from build123d import *

# Parameters (mm, degrees)
EXTRUDE_1_DEPTH     = 200
SKETCH_2_W          = 148
SKETCH_2_H          = 194
CUT_EXTRUDE_1_DEPTH = 44
SKETCH_3_W          = 9
SKETCH_3_H          = 194
EXTRUDE_1_2_DEPTH   = 44
CUT_EXTRUDE_2_DEPTH = 222.580685079
CUT_EXTRUDE_3_DEPTH = 219.876677606


with BuildPart() as part:
    # 草图1 → Extrude 1 (new body)
    with BuildSketch(Plane.XY):
        Polygon((77, 0), (-77, 0), (-77, 31), (-83, 37), (-83, 41), (-77, 47), (77, 47), (83, 41), (83, 37), (77, 31), align=None)
    extrude(amount=-EXTRUDE_1_DEPTH)

    # 草图2 → 切除-拉伸1 (cut)
    with BuildSketch(Plane(origin=(0, 47, 0), x_dir=(1, 0, 0), z_dir=(0, 1, 0))):
        with Locations((0, 100)):
            Rectangle(SKETCH_2_W, SKETCH_2_H)
    extrude(amount=-CUT_EXTRUDE_1_DEPTH, mode=Mode.SUBTRACT)

    # 草图3 → Extrude 1 2 (add)
    with BuildSketch(Plane(origin=(0, 3, 0), x_dir=(1, 0, 0), z_dir=(0, 1, 0))):
        with Locations((1.5, 100)):
            Rectangle(SKETCH_3_W, SKETCH_3_H)
    extrude(amount=EXTRUDE_1_2_DEPTH)

    # 草图5 → 切除-拉伸2 (cut, through all)
    with BuildSketch(Plane(origin=(0, 0, -200), x_dir=(-1, 0, 0), z_dir=(0, 0, -1))):
        Polygon((-74, 47), (-74, 44.343145751), (-79, 39.343145751), (-79, 38.656854249), (-74, 33.656854249), (-74, 23), (-6, 23), (-6, 32.656854249), (0, 38.656854249), (0, 39.343145751), (-4.7940469, 44.137192651), (-4.7940469, 47), align=None)
    extrude(amount=-CUT_EXTRUDE_2_DEPTH, mode=Mode.SUBTRACT)

    # 草图6 → 切除-拉伸3 (cut, through all)
    with BuildSketch(Plane(origin=(0, 0, -3), x_dir=(-1, 0, 0), z_dir=(0, 0, -1))):
        Polygon((-4.828427125, 47), (3, 47), (74, 47), (74, 39.171572875), (3, 39.171572875), align=None)
    extrude(amount=CUT_EXTRUDE_3_DEPTH, mode=Mode.SUBTRACT)


solid = part.part
The model under review builds one solid part; all positions refer to its coordinate system, in mm. A direction names the side the tool comes from. Give positions to 0.01 mm unless a question says otherwise; leave off trailing zeros. Order: outer loops, then holes, each group sorted by start corner. A loop starts at its lowest first (then second) coordinate and runs counter-clockwise, first axis right, second up. Notation, with made-up numbers: M 55,53 L 79,53 A15 ccw 79,77 Z; hole C -3.75,83.5 d7. An arc over 180 degrees is marked long. Answer in a Markdown table with one row per item. Add a question column.
1. Add section A-A on y = 26.5. State the section outline as (x, z) points.
2. For pin 1 Ø21.5 at (x, z) = (-21.5, -84.5) entering from +Y; pin 2 Ø0.9 at (x, z) = (34.5, -2) entering from +Y; pin 3 Ø1.5 at (y, z) = (6, -139.5) entering from +X, all flat-tipped, find the tip position at first contact; note any pin that passes through.
3. Add section D-D on z = -24. State the section outline as (x, y) points.
4. Machinability: for faces 5 (the flat face through (3.042, 35.615, -101.4)), 6 (the flat face through (40, 3, -101)), 7 (the flat face through (77, 16, -99)), which of the approach directions +Z, -Z, +X, -X, +Y, -Y give a long, thin tool a straight path to every point of the face, cutting with its end or side? Answer none if there is none.
5. Add section B-B on y = 8. State the section outline as (x, z) points.
6. Mouldability with a two-part tool opening along Z and no side actions: class faces 1 (the flat face through (1, 19, -200)), 2 (the flat face through (40, 13, -197)), 3 (the flat face through (-80, 44, -99)), 4 (the flat face through (-35, 25, -3)) as released by +Z, released by -Z, zero draft, split by the parting line, or undercut.
7. To check wall thickness, follow line 1 along X through (y, z) = (10, -90); line 2 along X through (y, z) = (33.5, -60); line 3 along Z through (x, y) = (58, 18). State the ranges of each line that lie inside material, in increasing order.
8. Add section C-C on x = -63.5. State the section outline as (y, z) points, plus the area to 3 significant figures.
The answers:
| question | item | result |
|---|---|---|
| 1 | outline | M -77,-200 L 6,-200 L 6,0 L -77,0 Z; M 74,-200 L 77,-200 L 77,0 L 74,0 Z; hole M -74,-197 L -3,-197 L -3,-3 L -74,-3 Z |
| 2 | pin 1 | y = 3 |
| 2 | pin 2 | y = 23 |
| 2 | pin 3 | x = 77 |
| 3 | outline | M -83,37 L -77,31 L -77,0 L 77,0 L 77,31 L 83,37 L 83,41 L 77,47 L 74,47 L 74,44.34 L 79,39.34 L 79,38.66 L 74,33.66 L 74,3 L 6,3 L 6,32.66 L 0,38.66 L 0,39.34 L 4.79,44.14 L 4.79,46.97 L -3,39.17 L -3,3 L -74,3 L -74,47 L -77,47 L -83,41 Z |
| 4 | face 5 | +Z, -Z |
| 4 | face 6 | +Y |
| 4 | face 7 | +Z, -Z, +X, -Y |
| 5 | outline | M -77,-200 L 77,-200 L 77,0 L -77,0 Z; hole M -74,-197 L -3,-197 L -3,-3 L -74,-3 Z; hole M 6,-197 L 74,-197 L 74,-3 L 6,-3 Z |
| 6 | face 1 | released by -Z |
| 6 | face 2 | undercut |
| 6 | face 3 | zero draft |
| 6 | face 4 | undercut |
| 7 | line 1 | -77 to -74, -3 to 6, 74 to 77 |
| 7 | line 2 | -79.5 to -74, -3 to 5.16, 74 to 79.5 |
| 7 | line 3 | -200 to -197, -3 to 0 |
| 8 | outline | M 0,-200 L 39.17,-200 L 39.17,-197 L 3,-197 L 3,-3 L 47,-3 L 47,0 L 0,0 Z |
| 8 | area | 841 mm2 |
